```python
from build123d import *

# Parameters (mm, degrees)
SKETCH1_W                      = 140
SKETCH1_H                      = 70
BASE_FLANGE1_DEPTH             = 1
EDGE_FLANGE1_STRIP_W           = 6
EDGE_FLANGE1_STRIP_H           = 1
EDGE_FLANGE1_STRIP_CUT_DEPTH   = 140
EDGE_FLANGE1_STRIP_2_W         = 6
EDGE_FLANGE1_STRIP_2_H         = 1
EDGE_FLANGE1_STRIP_CUT_2_DEPTH = 140
EDGE_FLANGE1_DEPTH             = 140
EDGE_FLANGE1_BEND_DEPTH        = 140
EDGE_FLANGE2_STRIP_W           = 6
EDGE_FLANGE2_STRIP_H           = 1
EDGE_FLANGE2_STRIP_CUT_DEPTH   = 140
EDGE_FLANGE2_DEPTH             = 140
EDGE_FLANGE3_STRIP_W           = 6
EDGE_FLANGE3_STRIP_H           = 1
EDGE_FLANGE3_STRIP_CUT_DEPTH   = 140
EDGE_FLANGE3_DEPTH             = 140
CUT_EXTRUDE1_DEPTH             = 120.783137378
CUT_EXTRUDE1_DEPTH_BACK        = 120.783137378
SKETCH18_W                     = 2
SKETCH18_H                     = 20
CUT_EXTRUDE2_DEPTH             = 101.56341283
CUT_EXTRUDE2_DEPTH_BACK        = 101.56341283
SKETCH20_R                     = 2.651793261
CUT_EXTRUDE3_DEPTH             = 102.143462468
CUT_EXTRUDE3_DEPTH_BACK        = 102.143462468
SKETCH21_R                     = 4.568960442


# Sheet-metal steps are written as plain solids
with BuildPart() as part:
    # Sketch1 → Base-Flange1 (new body)
    with BuildSketch(Plane(origin=(0, 0, 0), x_dir=(1, 0, 0), z_dir=(0, 1, 0))):
        Rectangle(SKETCH1_W, SKETCH1_H)
    extrude(amount=-BASE_FLANGE1_DEPTH)

    # Edge-Flange1 strip (across the edge) → Edge-Flange1 strip cut (cut)
    with BuildSketch(Plane(origin=(-70, 0, 35), x_dir=(0, 0, -1), z_dir=(1, 0, 0))):
        with Locations((-1, -0.5)):
            Rectangle(EDGE_FLANGE1_STRIP_W, EDGE_FLANGE1_STRIP_H)
    extrude(amount=EDGE_FLANGE1_STRIP_CUT_DEPTH, mode=Mode.SUBTRACT)

    # Edge-Flange1 strip 2 (across the edge) → Edge-Flange1 strip cut 2 (cut)
    with BuildSketch(Plane(origin=(70, 0, -35), x_dir=(0, 0, 1), z_dir=(-1, 0, 0))):
        with Locations((-1, -0.5)):
            Rectangle(EDGE_FLANGE1_STRIP_2_W, EDGE_FLANGE1_STRIP_2_H)
    extrude(amount=EDGE_FLANGE1_STRIP_CUT_2_DEPTH, mode=Mode.SUBTRACT)

    # Edge-Flange1 section (across the edge) → Edge-Flange1 (add)
    with BuildSketch(Plane(origin=(-70, 0, 35), x_dir=(0, 0, -1), z_dir=(1, 0, 0))):
        with BuildLine():
            Line((0, 1), (0, 58))
            Line((0, 58), (1, 58))
            Line((1, 58), (1, 1))
            ThreePointArc((1, 1), (1.292893219, 0.292893219), (2, 0))
            Line((2, 0), (2, -1))
            ThreePointArc((2, -1), (0.585786438, -0.414213562), (0, 1))
        make_face()
    extrude(amount=EDGE_FLANGE1_DEPTH)

    # Edge-Flange1 section 2 (across the edge) → Edge-Flange1 bend (add)
    with BuildSketch(Plane(origin=(70, 0, -35), x_dir=(0, 0, 1), z_dir=(-1, 0, 0))):
        with BuildLine():
            Line((0, 1), (0, 58))
            Line((0, 58), (1, 58))
            Line((1, 58), (1, 1))
            ThreePointArc((1, 1), (1.292893219, 0.292893219), (2, 0))
            Line((2, 0), (2, -1))
            ThreePointArc((2, -1), (0.585786438, -0.414213562), (0, 1))
        make_face()
    extrude(amount=EDGE_FLANGE1_BEND_DEPTH)

    # Edge-Flange2 strip (across the edge) → Edge-Flange2 strip cut (cut)
    with BuildSketch(Plane(origin=(70, 58, 35), x_dir=(0, -1, 0), z_dir=(-1, 0, 0))):
        with Locations((-1, -0.5)):
            Rectangle(EDGE_FLANGE2_STRIP_W, EDGE_FLANGE2_STRIP_H)
    extrude(amount=EDGE_FLANGE2_STRIP_CUT_DEPTH, mode=Mode.SUBTRACT)

    # Edge-Flange2 section (across the edge) → Edge-Flange2 (add)
    with BuildSketch(Plane(origin=(70, 58, 35), x_dir=(0, -1, 0), z_dir=(-1, 0, 0))):
        with BuildLine():
            Line((0, 1), (0, 8))
            Line((0, 8), (1, 8))
            Line((1, 8), (1, 1))
            ThreePointArc((1, 1), (1.292893219, 0.292893219), (2, 0))
            Line((2, 0), (2, -1))
            ThreePointArc((2, -1), (0.585786438, -0.414213562), (0, 1))
        make_face()
    extrude(amount=EDGE_FLANGE2_DEPTH)

    # Edge-Flange3 strip (across the edge) → Edge-Flange3 strip cut (cut)
    with BuildSketch(Plane(origin=(-70, 58, -35), x_dir=(0, -1, 0), z_dir=(1, 0, 0))):
        with Locations((-1, -0.5)):
            Rectangle(EDGE_FLANGE3_STRIP_W, EDGE_FLANGE3_STRIP_H)
    extrude(amount=EDGE_FLANGE3_STRIP_CUT_DEPTH, mode=Mode.SUBTRACT)

    # Edge-Flange3 section (across the edge) → Edge-Flange3 (add)
    with BuildSketch(Plane(origin=(-70, 58, -35), x_dir=(0, -1, 0), z_dir=(1, 0, 0))):
        with BuildLine():
            Line((0, 1), (0, 8))
            Line((0, 8), (1, 8))
            Line((1, 8), (1, 1))
            ThreePointArc((1, 1), (1.292893219, 0.292893219), (2, 0))
            Line((2, 0), (2, -1))
            ThreePointArc((2, -1), (0.585786438, -0.414213562), (0, 1))
        make_face()
    extrude(amount=EDGE_FLANGE3_DEPTH)

    # Sketch18 → Cut-Extrude1 (cut, two sides: drawn at the far end of the back side and taken through both)
    with BuildSketch(Plane.XY.offset(35).offset(-CUT_EXTRUDE1_DEPTH_BACK)):
        with Locations((-42.587057136, 22.971771136)):
            Rectangle(SKETCH18_W, SKETCH18_H)
        with Locations((-52.587057136, 22.971771136)):
            Rectangle(SKETCH18_W, SKETCH18_H)
        with Locations((-32.587057136, 22.971771136)):
            Rectangle(SKETCH18_W, SKETCH18_H)
        with Locations((-22.587057136, 22.971771136)):
            Rectangle(SKETCH18_W, SKETCH18_H)
        with Locations((-12.587057136, 22.971771136)):
            Rectangle(SKETCH18_W, SKETCH18_H)
        with Locations((-2.587057136, 22.971771136)):
            Rectangle(SKETCH18_W, SKETCH18_H)
        with Locations((7.412942864, 22.971771136)):
            Rectangle(SKETCH18_W, SKETCH18_H)
        with Locations((17.412942864, 22.971771136)):
            Rectangle(SKETCH18_W, SKETCH18_H)
        with Locations((27.412942864, 22.971771136)):
            Rectangle(SKETCH18_W, SKETCH18_H)
        with Locations((37.412942864, 22.971771136)):
            Rectangle(SKETCH18_W, SKETCH18_H)
        with Locations((47.412942864, 22.971771136)):
            Rectangle(SKETCH18_W, SKETCH18_H)
    extrude(amount=CUT_EXTRUDE1_DEPTH + CUT_EXTRUDE1_DEPTH_BACK, mode=Mode.SUBTRACT)

    # Sketch20 → Cut-Extrude2 (cut, two sides: drawn at the far end of the back side and taken through both)
    with BuildSketch(Plane.XZ.offset(-57).offset(-CUT_EXTRUDE2_DEPTH_BACK)):
        with Locations(Location((-55.216327322, 39.5, 0), (0, 0, 270))):
            Circle(SKETCH20_R)
        with Locations(Location((-55.216327322, -39.5, 0), (0, 0, 270))):
            Circle(SKETCH20_R)
        with Locations(Location((55.216327322, -39.5, 0), (0, 0, 270))):
            Circle(SKETCH20_R)
        with Locations(Location((55.216327322, 39.5, 0), (0, 0, 270))):
            Circle(SKETCH20_R)
    extrude(amount=CUT_EXTRUDE2_DEPTH + CUT_EXTRUDE2_DEPTH_BACK, mode=Mode.SUBTRACT)

    # Sketch21 → Cut-Extrude3 (cut, two sides: drawn at the far end of the back side and taken through both)
    with BuildSketch(Plane.XZ.offset(1).offset(-CUT_EXTRUDE3_DEPTH_BACK)):
        with Locations(Location((52.700809146, 16.902528803, 0), (0, 0, 270))):
            Circle(SKETCH21_R)
        with Locations(Location((52.700809146, -16.902528803, 0), (0, 0, 270))):
            Circle(SKETCH21_R)
    extrude(amount=CUT_EXTRUDE3_DEPTH + CUT_EXTRUDE3_DEPTH_BACK, mode=Mode.SUBTRACT)


solid = part.part
```
Work out the finished part from the listing and answer in its coordinate system (mm). A direction names the side the tool comes from. Round coordinates to 2 decimals unless told otherwise and drop trailing zeros. Loops run counter-clockwise (first coordinate to the right, second up) from the corner with the lowest first, then second, coordinate; pieces in that order, holes last. Notation, with made-up numbers: M 59,55 L 108,55 A10 cw 108,63 Z; hole C 22,-29 d10. An arc over 180 degrees is marked long. Use CSV: the item, a comma, the result in double quotes.
Q1. Section C-C, the plane x = 42 is taken. Determine the outline of the cut face in (y, z).
Determined:
outline,"M -1,-33 A2 ccw 1,-35 L 56,-35 A1 cw 57,-36 L 57,-43 L 58,-43 L 58,-36 A2 ccw 56,-34 L 1,-34 A1 cw 0,-33 L 0,33 A1 cw 1,34 L 56,34 A2 ccw 58,36 L 58,43 L 57,43 L 57,36 A1 cw 56,35 L 1,35 A2 ccw -1,33 Z"
Q2. Section D-D, the plane y = 30.5 is taken. State how many separate pieces and enclosed holes the cut face has, then the cut area to 3 significant figures.
Determined:
separate pieces,"24"
enclosed holes,"0"
area,"236 mm2"
Q3. The mould has two halves that part along Z. Classify faces 1 (the flat face through (-1, 28, 35)), 2 (the flat face through (-1, 0, 0)), 3 (the flat face through (1, 58, 39)): pulls with the +Z half, pulls with the -Z half, needs draft (parallel to the pull), parting line crosses it, or undercut.
Determined:
face 1,"pulls with the +Z half"
face 2,"undercut"
face 3,"needs draft"
Q4. A tool of negligible diameter and unlimited length cuts with its end or side. For faces 4 (the flat face through (-1, 58, -39)), 5 (the cylindrical face through (57.23, -0.49, 17.5)), 6 (the flat face through (1, 28, -35)), 7 (the flat face through (1, 29, -34)), 8 (the flat face through (1, 57, 40)), from which of +Z, -Z, +X, -X, +Y, -Y can it reach the whole face along a straight path? Write none if from no direction.
Determined:
face 4,"+Z, -Z, +X, -X, +Y"
face 5,"+Y, -Y"
face 6,"-Z, +X, -X, -Y"
face 7,"+X, -X, +Y"
face 8,"+Z, +X, -X, -Y"
Q5. Consider L1, parallel to X at y = 57.55, z = 39.5; L2, parallel to Z at x = -40, y = 9; L3, parallel to Y at x = -36, z = -11. Determine where each line is inside the solid, lowest interval first.
Determined:
L1,"-70 to -57.87, -52.56 to 52.56, 57.87 to 70"
L2,"-35 to -34, 34 to 35"
L3,"-1 to 0"
Q6. Section A-A, the plane y = 7.5 is taken. Determine the outline of the cut face in (x, z), then the cut area to 3 significant figures.
Determined:
outline,"M -70,-35 L 70,-35 L 70,-34 L -70,-34 Z; M -70,34 L 70,34 L 70,35 L -70,35 Z"
area,"280 mm2"
Q7. Section B-B, the plane z = 39.5 is taken. Determine the outline of the cut face in (x, y), then the cut area to 3 significant figures.
Determined:
outline,"M -70,57 L -57.87,57 L -57.87,58 L -70,58 Z; M -52.56,57 L 52.56,57 L 52.56,58 L -52.56,58 Z; M 57.87,57 L 70,57 L 70,58 L 57.87,58 Z"
area,"129 mm2"
Q8. Each of these flat-tipped pins is pushed along its axis until it touches: pin 1 (2 mm diameter, centred on x = -31.5, y = 40.5, fed in from -Z); pin 2 (1.1 mm diameter, centred on x = -53, z = -34.5, fed in from +Y); pin 3 (7 mm diameter, centred on x = -55.22, z = -39.5, fed in from -Y). Where does it stop, or does it pass through?
Determined:
pin 1,"z = -35"
pin 2,"y = 57.76"
pin 3,"y = 57"
